```python
from build123d import *

# Parameters (mm, degrees)
BOSS_EXTRUDE1_DEPTH = 12.7
FILLET1_R           = 3.175
FILLET2_R           = 1.5875
SKETCH2_R           = 2.45745
CUT_EXTRUDE1_DEPTH  = 13.7
SKETCH3_R           = 6.35
CUT_EXTRUDE2_DEPTH  = 2.54


with BuildPart() as part:
    # Sketch1 → Boss-Extrude1 (new body)
    with BuildSketch(Plane(origin=(0, 0, 0), x_dir=(1, 0, 0), z_dir=(0, 1, 0))):
        Polygon((-25.4, 0), (25.4, 0), (25.4, 95.25), (1.651, 95.25), (1.651, 44.45), (-1.651, 44.45), (-1.651, 95.25), (-25.4, 95.25), align=None)
    extrude(amount=BOSS_EXTRUDE1_DEPTH)

    # Fillet1
    fillet1_edges = [part.edges().sort_by_distance(p)[0] for p in [
        (-25.4, 6.35, -95.25),
        (-1.651, 6.35, -95.25),
        (1.651, 6.35, -95.25),
        (25.4, 6.35, -95.25),
        (25.4, 6.35, 0),
        (-25.4, 6.35, 0),
    ]]
    fillet(fillet1_edges, radius=FILLET1_R)

    # Fillet2
    fillet2_edges = [part.edges().sort_by_distance(p)[0] for p in [
        (-1.651, 6.35, -44.45),
        (1.651, 6.35, -44.45),
    ]]
    fillet(fillet2_edges, radius=FILLET2_R)

    # Sketch2 → Cut-Extrude1 (cut, through all)
    with BuildSketch(Plane.XZ):
        with Locations((-12.7, -36.7538)):
            Circle(SKETCH2_R)
        with Locations((12.7, -36.7538)):
            Circle(SKETCH2_R)
    extrude(amount=-CUT_EXTRUDE1_DEPTH, mode=Mode.SUBTRACT)

    # Sketch3 → Cut-Extrude2 (cut)
    with BuildSketch(Plane(origin=(0, 12.7, 0), x_dir=(1, 0, 0), z_dir=(0, 1, 0))):
        with Locations((12.7, 36.7538)):
            Circle(SKETCH3_R)
        with Locations((-12.7, 36.7538)):
            Circle(SKETCH3_R)
    extrude(amount=-CUT_EXTRUDE2_DEPTH, mode=Mode.SUBTRACT)


solid = part.part
```
Design review of the part built by this model. Coordinates are the model's own, in mm. A direction names the side the tool comes from. Round coordinates to 2 decimals unless told otherwise and drop trailing zeros. Write each loop counter-clockwise with the first axis right and the second up, starting at its lowest first coordinate (ties: lowest second). Pieces come first, ordered by that corner, then holes.
Item 1: We need section A-A on z = -78.5. Write out the cut boundary in (x, y).
Item 2: We need section C-C on y = 3.25. State how many separate pieces and enclosed holes the cut face has, and give its area (3 significant figures).
Item 3: We need section B-B on x = 12.7. Write out the cut boundary in (y, z).
Item 4: Clearance check with flat-ended pins moving along their axes: pin 1 Ø14.5 at (x, z) = (12.7, -36.75) entering from -Y; pin 2 Ø4 at (x, z) = (-11, -39.5) entering from +Y; pin 3 Ø4.5 at (x, z) = (12.7, -36.75) entering from +Y. State where each tip first meets the part, or that it passes through.
Item 5: For probe 1 along X at (y, z) = (9, -58.5); probe 2 along Z at (x, y) = (12.7, 4.5); probe 3 along Z at (x, y) = (-12.7, 11.45), list the stretches that pass through material, from the lowest coordinate up.
Item 6: The part is to be moulded in two halves that separate along Z. For faces 1 (the cylindrical face through (-2.56, 6.44, -94.3)), 2 (the flat face through (0, 6, 0)), 3 (the cylindrical face through (13.834, 5.009, -38.934)), say which applies: +Z half, -Z half, draft (parallel to the pull), parting line (faces both ways), or undercut.
Item 7: We need section D-D on z = -42. Write out the cut boundary in (x, y).
Item 8: For faces 4 (the cylindrical face through (-24.45, 6.44, -94.34)), 5 (the flat face through (1.651, 6, -69)), 6 (the flat face through (15.4, 10.16, -36.8)), list the 3-axis set-ups (+Z, -Z, +X, -X, +Y, -Y) from which the entire face can be reached by the end or side of a thin tool; tool diameter is ignored.
Returned:
1. outline: (-25.4, 0) - (-1.65, 0) - (-1.65, 12.7) - (-25.4, 12.7) - close; (1.65, 0) - (25.4, 0) - (25.4, 12.7) - (1.65, 12.7) - close
2. separate pieces: 1
2. enclosed holes: 2
2. area: 4,620 mm2
3. outline: (0, -95.25) - (12.7, -95.25) - (12.7, -43.1) - (10.16, -43.1) - (10.16, -39.21) - (0, -39.21) - close; (0, -34.3) - (10.16, -34.3) - (10.16, -30.4) - (12.7, -30.4) - (12.7, 0) - (0, 0) - close
4. pin 1: stops at y = 0
4. pin 2: stops at y = 10.16
4. pin 3: passes through
5. probe 1: x = -25.4 to -1.65, 1.65 to 25.4
5. probe 2: z = -95.25 to -39.21, -34.3 to 0
5. probe 3: z = -95.25 to -43.1, -30.4 to 0
6. face 1: -Z half
6. face 2: +Z half
6. face 3: undercut
7. outline: (-25.4, 0) - (25.4, 0) - (25.4, 12.7) - (16.28, 12.7) - (16.28, 10.16) - (9.12, 10.16) - (9.12, 12.7) - (-9.12, 12.7) - (-9.12, 10.16) - (-16.28, 10.16) - (-16.28, 12.7) - (-25.4, 12.7) - close
8. face 4: -Z, -X, +Y, -Y
8. face 5: -Z, +Y, -Y
8. face 6: +Y
